Autodesk Inventor part; units mm, degrees
ref_plane "Work Plane1" through (-30.481, -38.481, 0) normal (-1, 0, 0) x (0, 0, 1)
ref_plane "Work Plane2" through (-38.481, -30.481, 0) normal (0, -1, 0) x (1, 0, 0)
ref_plane "YZ Plane" through (0, 0, 0) normal (1, 0, 0) x (0, 1, 0)
sketch "Sketch1" plane through (0, 0, 0) normal (0, 0, 1) x (1, 0, 0)
  line L0 (-38.481, 38.481) -> (38.481, 38.481)
  line L1 (38.481, 38.481) -> (38.481, -38.481)
  line L2 (38.481, -38.481) -> (-38.481, -38.481)
  line L3 (-38.481, -38.481) -> (-38.481, 38.481)
  point P0 (0, 0)
  dimension "d0" = 76.962
  dimension "d1" = 76.962
  dimension "d2" = 38.481
  dimension "d3" = 38.481
extrude "Extrusion1" add sketch "Sketch1" against normal blind 25.4
sketch "Sketch2" plane through (0, 0, 0) normal (0, 0, 1) x (1, 0, 0)
  line L0 (-38.481, 38.481) -> (38.481, 38.481)
  line L1 (-38.481, -38.481) -> (-38.481, 38.481)
  line L2 (38.481, -38.481) -> (-38.481, -38.481)
  line L3 (38.481, 38.481) -> (38.481, -38.481)
  line L4 (-30.481, 38.481) -> (-30.481, 28.481)
  line L5 (-30.481, 28.481) -> (28.481, -30.481)
  line L6 (28.481, -30.481) -> (38.481, -30.481)
  line L7 (-30.481, 17.1673) -> (-30.481, -30.481)
  line L8 (-30.481, -30.481) -> (17.1673, -30.481)
  line L9 (17.1673, -30.481) -> (-30.481, 17.1673)
  dimension "d6" = 8
  dimension "d7" = 8
  dimension "d8" = 10
  dimension "d10" = 135
  dimension "d11" = 8
extrude "Extrusion2" cut sketch "Sketch2" against normal through all contours L0 L3 L6 L5 L4 | L9 L8 L7
fillet "Fillet1" radius 2 1 edges at (-30.481, -30.481, -12.7)
fillet "Fillet1" radius 1 4 edges at (-30.481, 38.481, -12.7) (-30.481, 28.481, -12.7) (28.481, -30.481, -12.7) (38.481, -30.481, -12.7)
fillet "Fillet1" radius 3 2 edges at (-30.481, 17.1673, -12.7) (17.1673, -30.481, -12.7)
sketch "Sketch3" plane through (-38.481, -38.481, 0) normal (-1, 0, 0) x (0, 0, 1)
  line L0 (0, 0) -> (-25.4, 0)
  line L1 (0, 0) -> (0, 76.962)
  point P0 (-12.7, 60)
  point P1 (-12.7, 20)
  dimension "d17" = 12.7
  dimension "d18" = 20
  dimension "d19" = 40
hole "Hole1" at (-38.481, 21.519, -12.7) at (-38.481, -18.481, -12.7) direction (1, 0, 0) diameter 7 end through all
sketch "Sketch4" plane through (-38.481, -38.481, 0) normal (0, -1, 0) x (1, 0, 0)
  line L0 (0, -25.4) -> (76.962, -25.4)
  line L1 (0, 0) -> (0, -25.4)
  point P0 (20, -12.7)
  point P1 (60, -12.7)
  dimension "d27" = 12.7
  dimension "d28" = 20
  dimension "d29" = 40
hole "Hole2" at (-18.481, -38.481, -12.7) at (21.519, -38.481, -12.7) direction (0, 1, 0) diameter 7 end through all
ref_plane "Work Plane1" through (-30.481, -38.481, 0) normal (-1, 0, 0) x (0, 0, 1)
ref_plane "Work Plane2" through (-38.481, -30.481, 0) normal (0, -1, 0) x (1, 0, 0)
sketch "Sketch5" plane through (-30.481, -38.481, 0) normal (-1, 0, 0) x (0, 0, 1)
  arc A0 (-15.1299, 57.481) -> (-10.2701, 57.481) centre (-12.7, 60) ccw
  arc A1 (-10.2701, 57.481) -> (-15.1299, 57.481) centre (-12.7, 60) ccw
  circle A2 centre (-12.7, 60) radius 3.5
  circle A3 centre (-12.7, 60) radius 6
  dimension "d39" = 12
extrude "Extrusion3" cut sketch "Sketch5" against normal through all
sketch "Sketch6" plane through (-38.481, -30.481, 0) normal (0, -1, 0) x (1, 0, 0)
  arc A0 (57.481, -10.2701) -> (57.481, -15.1299) centre (60, -12.7) ccw
  arc A1 (57.481, -15.1299) -> (57.481, -10.2701) centre (60, -12.7) ccw
  circle A2 centre (60, -12.7) radius 3.5
  circle A3 centre (60, -12.7) radius 6
  dimension "d42" = 12
extrude "Extrusion4" cut sketch "Sketch6" against normal through all
ref_plane "OffsetPlane" through (0, 0, -12.7) normal (0, 0, 1) x (1, 0, 0)
properties part number "20-101" material "Alluminio - 6061"
Input: part model. Units: mm. Frame: model coordinates. A direction names the side the tool comes from. Give positions to 0.01 mm unless a question says otherwise; leave off trailing zeros. Order: outer loops, then holes, each group sorted by start corner. A loop starts at its lowest first (then second) coordinate and runs counter-clockwise, first axis right, second up. Notation, with made-up numbers: (84, -0.75) - (109, -0.75) arc R18 ccw to (109, 5.25) - close; hole circle Ø1 at (6, 89.25). An arc over 180 degrees is marked (long way). Answer as a JSON object with one key per item and string values. Group by question number.
Q1. Cut plane C-C, the plane x = 23. Output: boundary loops of the cut face in (y, z), then the cut area to 3 significant figures.
Q2. Cut plane A-A, the plane z = -23.5. Output: boundary loops of the cut face in (x, y).
Q3. First-contact query: pin 1 Ø4 at (x, z) = (-18.481, -12.7) entering from -Y; pin 2 Ø8 at (x, z) = (-18.481, -12.7) entering from +Y; pin 3 Ø12.5 at (x, z) = (-9.5, -16) entering from +Y; pin 4 Ø2.5 at (x, z) = (32.5, -13.5) entering from +Y. Flat tips, straight axial feed; report the tip coordinate or a pass-through.
Q4. Cut plane B-B, the plane y = 3. Output: boundary loops of the cut face in (x, z), then the cut area to 3 significant figures.
Q5. Mould query, pull axis X, two halves, no side actions, for faces 1 (the face through (-3, -8, -25.4)), 2 (the face through (-30.481, 19, -10)), 3 (the face through (-6.395, -6.919, -12.522)). Classes: pulls with the +X half, pulls with the -X half, needs draft (parallel to the pull), parting line crosses it, or undercut.
Q6. Line query: probe 1 along Y at (x, z) = (-33.25, -12.7); probe 2 along X at (y, z) = (10.5, -13.25); probe 3 along Y at (x, z) = (11, -12.25). Output: solid intervals per line, ascending.
Q7. Set-up query: faces 4 (the face through (24.1, -30.481, -15.3)), 5 (the face through (-25.96, 15.66, -14)), 6 (the face through (-29.88, -29.91, -12.88)), 7 (the face through (-30.481, 33, -13)). Return all of +Z, -Z, +X, -X, +Y, -Y with unobstructed straight access to the full face (end or side cutting, diameter ignored); none if empty.
Q8. Cut plane D-D, the plane x = -21. Output: boundary loops of the cut face in (y, z).
Results:
{
 "1": {"outline": "(-38.48, -25.4) - (-25, -25.4) - (-25, -18.51) - (-30.48, -18.51) - (-30.48, -15.87) - (-38.48, -15.87) - close; (-38.48, -9.53) - (-30.48, -9.53) - (-30.48, -6.89) - (-25, -6.89) - (-25, 0) - (-38.48, 0) - close", "area": "228 mm^2"},
 "2": {"outline": "(-38.48, -38.48) - (38.48, -38.48) - (38.48, -31.48) arc R1 ccw to (37.48, -30.48) - (28.9, -30.48) arc R1 cw to (28.19, -30.19) - (-30.19, 28.19) arc R1 cw to (-30.48, 28.9) - (-30.48, 37.48) arc R1 ccw to (-31.48, 38.48) - (-38.48, 38.48) - close; hole (-30.48, -28.48) arc R2 ccw to (-28.48, -30.48) - (9.92, -30.48) arc R3 ccw to (12.05, -25.36) - (-25.36, 12.05) arc R3 ccw to (-30.48, 9.92) - close"},
 "3": {"pin 1": "through", "pin 2": "y = 17.02", "pin 3": "y = 13.75", "pin 4": "y = -30.48"},
 "4": {"outline": "(-38.48, -25.4) - (-30.48, -25.4) - (-30.48, 0) - (-38.48, 0) - close; (-16.31, -25.4) - (-5, -25.4) - (-5, 0) - (-16.31, 0) - (-16.31, -9.95) arc R3.5 cw to (-16.31, -15.45) - close", "area": "485 mm^2"},
 "5": {"face 1": "needs draft", "face 2": "pulls with the +X half", "face 3": "undercut"},
 "6": {"probe 1": "-38.48 to -21.98, -14.98 to 18.02, 25.02 to 38.48", "probe 2": "-38.48 to -30.43, -23.81 to -21.94, -15.02 to -12.5", "probe 3": "-38.48 to -30.28, -24.31 to -21.95, -15.01 to -13"},
 "7": {"face 4": "+Y", "face 5": "+X", "face 6": "+Z, -Z", "face 7": "+Z, -Z, +X, +Y"},
 "8": {"outline": "(-38.48, -25.4) - (-30.48, -25.4) - (-30.48, -15.13) - (-38.48, -15.13) - close; (-38.48, -10.27) - (-30.48, -10.27) - (-30.48, 0) - (-38.48, 0) - close; (7.69, -25.4) - (19, -25.4) - (19, -18.15) arc R6 cw to (16.03, -15.13) - (7.69, -15.13) - close; (7.69, -10.27) - (16.03, -10.27) arc R6 cw to (19, -7.25) - (19, 0) - (7.69, 0) - close"}
}
